from build123d import *

# Parameters (mm, degrees)
F0_W     = 177.8
F0_H     = 127
F1_DEPTH = 50.8
F1_TAPER = 5
F4_DEPTH = 6.35
F5_R     = 9.525
F6_T     = 2.54
F7_D     = 5.334


with BuildPart() as f1:
    # F0 (on Top) → F1 (new body)
    with BuildSketch(Plane.XY):
        Rectangle(F0_W, F0_H)
    extrude(amount=F1_DEPTH, taper=F1_TAPER)

    # F3 (on face) → F4 (cut)
    with BuildSketch(Plane.XY.offset(50.8)):
        with BuildLine():
            ThreePointArc((8.8899883424, -53.9606030597), (-0.0143969403, -45.0850116576), (-8.8899883424, -53.9893969403))
            Line((-8.8899883424, -53.9893969403), (-8.867513666, -67.8673187242))
            ThreePointArc((-8.867513666, -67.8673187242), (0.0368716166, -76.7429101263), (8.9124630188, -67.8385248437))
            Line((8.9124630188, -67.8385248437), (8.8899883424, -53.9606030597))
        make_face()
    extrude(amount=-F4_DEPTH, mode=Mode.SUBTRACT)

    # F5
    f5_edges = [f1.edges().sort_by_distance(p)[0] for p in [
        (-86.677788, 61.277788, 25.4),
        (-86.677788, -61.277788, 25.4),
        (86.677788, 61.277788, 25.4),
        (86.677788, -61.277788, 25.4),
    ]]
    fillet(f5_edges, radius=F5_R)

    # F6
    f6_openings = [f1.faces().sort_by_distance(p)[0] for p in [
        (0, 0, 0),
    ]]
    offset(amount=F6_T, openings=f6_openings, kind=Kind.INTERSECTION)

    # F7 (through all)
    with Locations(Plane.XY.offset(50.8)):
        with Locations((0, -53.975)):
            Hole(F7_D / 2)


solid = f1.part
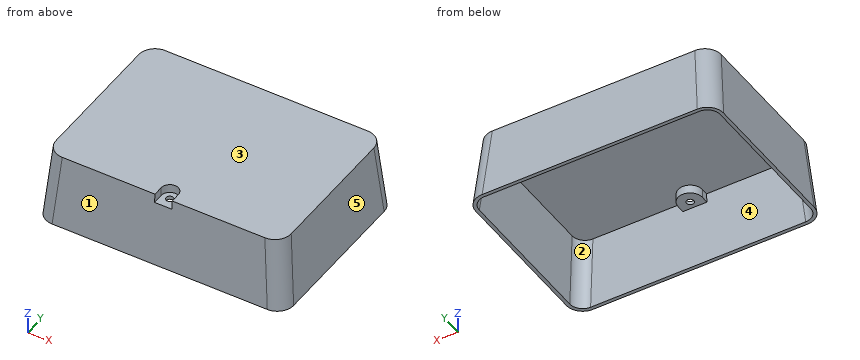
Part model, mm, in its own coordinate system. Face numbers are marked on the shaded views. A direction names the side the tool comes from. Coordinates: 2 decimals unless noted, no trailing zeros. Order: outer loops, then holes, each group sorted by start corner. A loop starts at its lowest first (then second) coordinate and runs counter-clockwise, first axis right, second up.
(1) Slice it at B-B, the plane y = -19. Write the cut outline in (x, z), and give its area (3 significant figures).
Check sheet entries:
outline: (-91.45, 0) - (-88.9, 0) - (-84.46, 50.8) - (84.46, 50.8) - (88.9, 0) - (91.45, 0) - (86.78, 53.34) - (-86.78, 53.34) - close
area: 700 mm2
(2) Slice it at A-A, the plane x = 0. Write the cut outline in (y, z) (3 decimals), and give its area (3 significant figures).
Check sheet entries:
outline: (-66.05, 0) - (-63.5, 0) - (-59.611, 44.45) - (-56.642, 44.45) - (-56.642, 46.99) - (-61.939, 46.99) - close; (-51.308, 44.45) - (-45.085, 44.45) - (-45.085, 50.8) - (59.056, 50.8) - (63.5, 0) - (66.05, 0) - (61.383, 53.34) - (-47.625, 53.34) - (-47.625, 46.99) - (-51.308, 46.99) - close
area: 559 mm2
(3) Probe L1, parallel to Y at x = 0, z = 46.2 (3 decimals); L2, parallel to Y at x = 0, z = 45 (3 decimals); L3, parallel to Z at x = 27.5, y = 21. List the from-to ranges inside material, lowest first.
Check sheet entries:
L1: y = -62.008 to -56.642, -51.308 to -45.085, 59.458 to 62.008
L2: y = -62.113 to -56.642, -51.308 to -45.085, 59.563 to 62.113
L3: z = 50.8 to 53.34
(4) Pull direction X, two halves, no side cores. Call the marked faces 3, 4 and 5: pulls with the +X half, pulls with the -X half, needs draft (parallel to the pull), parting line crosses it, or undercut.
Check sheet entries:
face 3: needs draft
face 4: undercut
face 5: pulls with the +X half
(5) Slice it at C-C, the plane x = -44.5. Write the cut outline in (y, z), and give its area (3 significant figures).
Check sheet entries:
outline: (-66.05, 0) - (-63.5, 0) - (-59.06, 50.8) - (59.06, 50.8) - (63.5, 0) - (66.05, 0) - (61.38, 53.34) - (-61.38, 53.34) - close
area: 571 mm2
(6) Pin check, flat tips, straight feed: pin 1 Ø5 at (y, z) = (50, 15) entering from -X; pin 2 Ø5 at (y, z) = (19.5, 44) entering from -X; pin 3 Ø6 at (x, y) = (0, -53.975) entering from +Z. Stop position of each tip, or through.
Check sheet entries:
pin 1: stops at x = -90.36
pin 2: stops at x = -87.82
pin 3: stops at z = 46.99
(7) Tool access for the marked faces 1 and 2: list every direction of +Z, -Z, +X, -X, +Y, -Y with a clear straight run to the whole face (end or side of a thin tool).
Check sheet entries:
face 1: +Z, +X, -X, -Y
face 2: -Z
